The model under review builds one solid part; all positions refer to its coordinate system, in mm. Face numbers are marked on the shaded views. A direction names the side the tool comes from. Coordinates: 2 decimals unless noted, no trailing zeros. Order: outer loops, then holes, each group sorted by start corner. A loop starts at its lowest first (then second) coordinate and runs counter-clockwise, first axis right, second up. Notation, with made-up numbers: M 67,40 L 124,40 A21 cw 124,51 Z; hole C -19.75,-33.75 d6. An arc over 180 degrees is marked long. One line per item, written item: value.
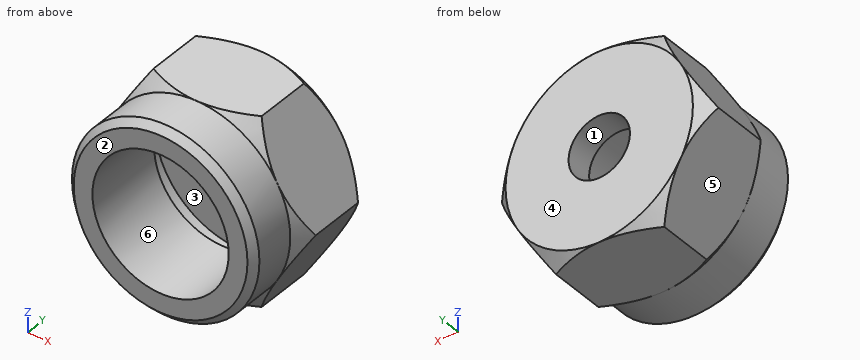
Autodesk Inventor part; units mm, degrees
ref_plane "Work Plane2" through (0, 12.5, 0) normal (0, -1, 0) x (1, 0, 0)
ref_plane "YZ Plane" through (0, 0, 0) normal (1, 0, 0) x (0, 1, 0)
ref_plane "XZ Plane" through (0, 0, 0) normal (0, 1, 0) x (-1, 0, 0)
sketch "Sketch4" plane through (0, 0, 0) normal (0, 1, 0) x (-1, 0, 0)
  line L0 (-31.7543, 0) -> (-15.8771, 27.5)
  line L1 (-15.8771, 27.5) -> (15.8771, 27.5)
  line L2 (15.8771, 27.5) -> (31.7543, 0)
  line L3 (31.7543, 0) -> (15.8771, -27.5)
  line L4 (15.8771, -27.5) -> (-15.8771, -27.5)
  line L5 (-15.8771, -27.5) -> (-31.7543, 0)
  line L6 (31.7543, 0) -> (-31.7543, 0)
  point P0 (0, 0)
  point P1 (0, 0)
extrude "Extrusion2" add sketch "Sketch4" along normal blind 25
sketch "Sketch12" plane through (0, 0, 0) normal (0, 0, 1) x (1, 0, 0)
  line L0 (-15.8771, 25) -> (-31.7543, 25)
  line L1 (-31.7543, 25) -> (-31.7543, 20.732)
  line L2 (-27.4862, 25) -> (-31.7543, 20.732)
  line L3 (0, -5) -> (0, 30)
  point P0 (0, 0)
  dimension "d23" = 45
revolve "Revolution1" cut sketch "Sketch12" angle 360 about axis through (0, -10, 0) along (0, 1, 0)
ref_plane "Work Plane2" through (0, 12.5, 0) normal (0, -1, 0) x (1, 0, 0)
mirror "Mirror1" about plane through (0, 12.5, 0) normal (0, -1, 0) of "Revolution1"
sketch "Sketch13" plane through (0, 25, 0) normal (0, 1, 0) x (1, 0, 0)
  circle A0 centre (0, 0) radius 9
  dimension "d25" = 18
extrude "Extrusion5" cut sketch "Sketch13" against normal blind 8
sketch "Sketch14" plane through (0, 17, 0) normal (0, 1, 0) x (1, 0, 0)
  circle A0 centre (0, 0) radius 25
  dimension "d28" = 50
extrude "Extrusion6" cut sketch "Sketch14" against normal blind 7
sketch "Sketch15" plane through (0, 0, 0) normal (0, -1, 0) x (1, 0, 0)
  circle A0 centre (0, 0) radius 27.5
  dimension "d32" = 55
extrude "Extrusion7" add sketch "Sketch15" along normal blind 14
sketch "Sketch16" plane through (0, 10, 0) normal (0, 1, 0) x (1, 0, 0)
  circle A0 centre (0, 0) radius 20
  dimension "d35" = 40
extrude "Extrusion8" cut sketch "Sketch16" against normal through all
chamfer "Chamfer1" distance 2 angle 45 1 edges at (-27.5, -14, 0)
thread "Thread2"
properties part number "00.32.007 \"Nut\"" material "Steel"
(1) Mouldability with a two-part tool opening along Y and no side actions: class the marked faces 1, 2, 3 and 4 as +Y half, -Y half, draft (parallel to the pull), parting line (faces both ways), or undercut.
Geometry results:
face 1: draft
face 2: -Y half
face 3: undercut
face 4: +Y half
(2) We need section D-D, the plane y = -7.5. State the section outline as (x, z) points, plus the area to 3 significant figures.
Geometry results:
outline: C 0,0 d55; hole C 0,0 d40
area: 1,120 mm2
(3) Tool access review of the marked faces 5 and 6: name each direction out of +Z, -Z, +X, -X, +Y, -Y from which nothing blocks a thin tool from reaching the whole face with its end or side.
Geometry results:
face 5: -Z, -X, +Y, -Y
face 6: -Y
(4) We need section B-B, the plane y = 11. State the section outline as (x, z) points.
Geometry results:
outline: M -31.75,0 L -15.88,-27.5 L 15.88,-27.5 L 31.75,0 L 15.88,27.5 L -15.88,27.5 Z; hole C 0,0 d50
(5) Insertion check: pin 1 Ø6 at (x, y) = (-12.5, -6) entering from +Z; pin 2 Ø2 at (y, z) = (-9, -11.5) entering from -X; pin 3 Ø3 at (x, y) = (-3.5, -7) entering from -Z. Each pin has a flat end and moves straight along its axis. Give the tip position at first contact, or say it passes through.
Geometry results:
pin 1: stops at z = 25.81
pin 2: stops at x = -25.42
pin 3: stops at z = -27.43
(6) For L1, parallel to Z at x = 0, y = 3; L2, parallel to Z at x = 0, y = 13.25; L3, parallel to Y at x = 21.5, z = -4, list the stretches that pass through material, from the lowest coordinate up.
Geometry results:
L1: z = -27.5 to -20, 20 to 27.5
L2: z = -27.5 to -25, 25 to 27.5
L3: y = -14 to 10, 17 to 25
(7) We need section C-C, the plane y = 18. State the section outline as (x, z) points.
Geometry results:
outline: M -31.75,0 L -15.88,-27.5 L 15.88,-27.5 L 31.75,0 L 15.88,27.5 L -15.88,27.5 Z; hole C 0,0 d18
